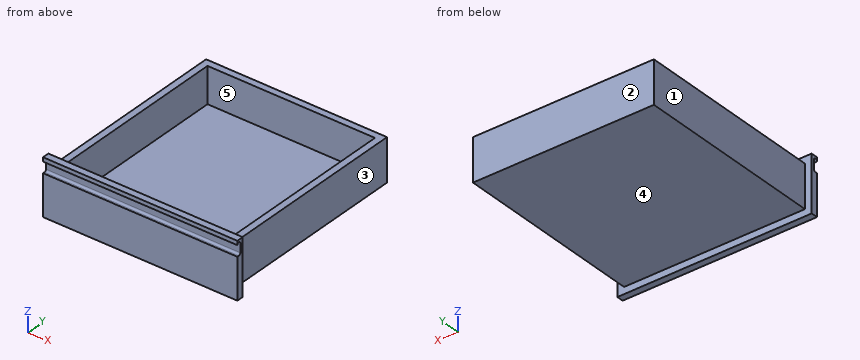
```python
from build123d import *

# Parameters (mm, degrees)
F0_W     = 520
F0_H     = 150
F0_W_2   = 484
F0_H_2   = 114
F1_DEPTH = 18
F2_DEPTH = 530
F3_W     = 448
F3_H     = 476
F4_DEPTH = 96
F6_DEPTH = 539


with BuildPart() as f1:
    # F0 (on Front) → F1 (new body)
    with BuildSketch(Plane.XZ):
        with Locations((260, 75)):
            Rectangle(F0_W, F0_H)
        with Locations((260, 75)):
            Rectangle(F0_W_2, F0_H_2, mode=Mode.SUBTRACT)
    extrude(amount=-F1_DEPTH)

    # F0 (on Front) → F2 (join)
    with BuildSketch(Plane.XZ):
        with Locations((260, 75)):
            Rectangle(F0_W_2, F0_H_2)
    extrude(amount=-F2_DEPTH)

    # F3 (on face) → F4 (cut)
    with BuildSketch(Plane.XY.offset(132)):
        with Locations((260, 274)):
            Rectangle(F3_W, F3_H)
    extrude(amount=-F4_DEPTH, mode=Mode.SUBTRACT)

    # F5 (on face) → F6 (cut)
    with BuildSketch(Plane(origin=(0, 0, 0), x_dir=(0, -1, 0), z_dir=(-1, 0, 0))):
        with BuildLine():
            Line((-5, 110), (0, 110))
            Line((0, 110), (0, 139))
            ThreePointArc((0, 139), (-5, 144), (-10, 139))
            Line((-10, 139), (-10, 115))
            ThreePointArc((-10, 115), (-8.535534, 111.464466), (-5, 110))
        make_face()
    extrude(amount=-F6_DEPTH, mode=Mode.SUBTRACT)


solid = f1.part
```
Input: part model. Units: mm. Frame: model coordinates. Face numbers are marked on the shaded views. A direction names the side the tool comes from. Give positions to 0.01 mm unless a question says otherwise; leave off trailing zeros. Loops run counter-clockwise (first coordinate to the right, second up) from the corner with the lowest first, then second, coordinate; pieces in that order, holes last. Notation, with made-up numbers: (18, 23.25) -> (36, 23.25) arc R28 cw to (36, 47.25) -> close; hole circle Ø8 at (-16, 53.25). An arc over 180 degrees is marked (long way). Use a Markdown table: item, result.
Q1. Section query B-B, the plane x = 313. Return the cut outline in (y, z).
Entries:
| item | result |
|---|---|
| outline | (0, 0) -> (18, 0) -> (18, 18) -> (530, 18) -> (530, 132) -> (512, 132) -> (512, 36) -> (36, 36) -> (36, 132) -> (18, 132) -> (18, 150) -> (0, 150) -> (0, 139) arc R5 cw to (10, 139) -> (10, 115) arc R5 cw to (5, 110) -> (0, 110) -> close |
Q2. Ray query, probe 1 along Y at (x, z) = (373, 88); probe 2 along X at (y, z) = (231.5, 59.5); probe 3 along Y at (x, z) = (37, 118). Return the intervals inside material, ascending. Write a range as from..to.
Entries:
| item | result |
|---|---|
| probe 1 | y = 0..36, 512..530 |
| probe 2 | x = 18..36, 484..502 |
| probe 3 | y = 10..36, 512..530 |
Q3. First-contact query: P1, Ø1, axis at x = 436.5, y = 455.5, coming from the -Z side; P2, Ø10, axis at x = 303.5, y = 323.5, coming from the +Z side; P3, Ø2, axis at y = 162.5, z = 73.5, coming from the -X side. Flat tips, straight axial feed; report the tip coordinate or a pass-through.
Entries:
| item | result |
|---|---|
| P1 | stops at z = 18 |
| P2 | stops at z = 36 |
| P3 | stops at x = 18 |
Q4. Section query C-C, the plane y = 357. Return the cut outline in (x, z).
Entries:
| item | result |
|---|---|
| outline | (18, 18) -> (502, 18) -> (502, 132) -> (484, 132) -> (484, 36) -> (36, 36) -> (36, 132) -> (18, 132) -> close |
Q5. Section query A-A, the plane z = 84. Return the cut outline in (x, y), plus the area to 3 significant figures.
Entries:
| item | result |
|---|---|
| outline | (0, 0) -> (520, 0) -> (520, 18) -> (502, 18) -> (502, 530) -> (18, 530) -> (18, 18) -> (0, 18) -> close; hole (36, 36) -> (484, 36) -> (484, 512) -> (36, 512) -> close |
| area | 43,900 mm² |
Q6. Access query for the marked faces 1, 2, 3, 4 and 5. Directions: +Z, -Z, +X, -X, +Y, -Y. A direction counts if a zero-diameter tool reaches every point of the face in a straight line with its end or side. Return the directions, or none.
Entries:
| item | result |
|---|---|
| face 1 | +Z, -Z, -X, +Y |
| face 2 | +Z, -Z, +X, -X, +Y |
| face 3 | +Z, -Z, +X, +Y |
| face 4 | -Z, +X, -X, +Y |
| face 5 | +Z |
